Source: three-view drawing plus pictorial views. Frame: mm from the lowest corner of the part. Give positions to 0.01 mm unless a question says otherwise; leave off trailing zeros. Order: outer loops, then holes, each group sorted by start corner. A loop starts at its lowest first (then second) coordinate and runs counter-clockwise, first axis right, second up. Notation, with made-up numbers: (-35, 22.25) -> (-13, 22.25) arc R13 ccw to (-13, 44.25) -> close; hole circle Ø4 at (85, -25). An arc over 180 degrees is marked (long way). Answer in a Markdown table with one row per item. Add a question column.
Q1. Cut plane A-A on x = 894.5. Return the cut outline in (y, z), and give its area (3 significant figures).
Q2. Cut plane C-C on z = 46. Return the cut outline in (x, y).
Q3. Cut plane B-B on y = 720. Return the cut outline in (x, z), and give its area (3 significant figures).
Q4. Contact query for a flat-ended pin moving along its axis: P1, Ø24, axis at x = 641.5, z = 68, coming from the -Y side. Output: stop coordinate, or through.
Q5. Line query: line 1 along X through (y, z) = (712, 72.5); line 2 along Y through (x, z) = (908, 79); line 3 along X through (y, z) = (195, 59). Output: solid intervals per line, ascending. Write a range as from..to.
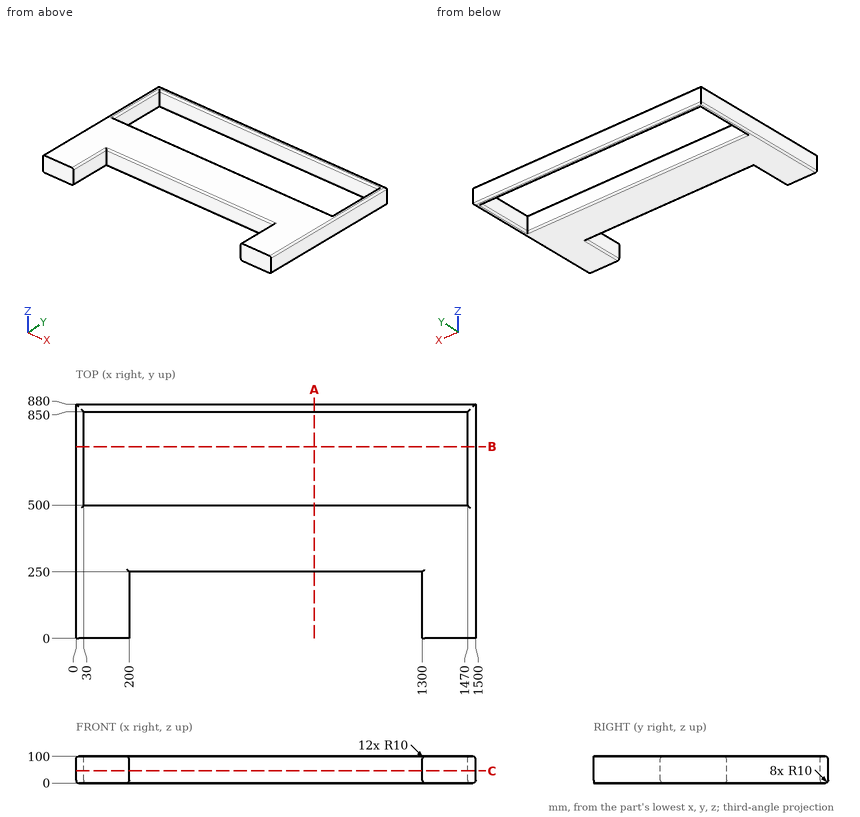
Completed:
| question | item | result |
|---|---|---|
| 1 | outline | (250, 10) arc R10 ccw to (260, 0) -> (490, 0) arc R10 ccw to (500, 10) -> (500, 90) arc R10 ccw to (490, 100) -> (260, 100) arc R10 ccw to (250, 90) -> close; (850, 10) arc R10 ccw to (860, 0) -> (870, 0) arc R10 ccw to (880, 10) -> (880, 90) arc R10 ccw to (870, 100) -> (860, 100) arc R10 ccw to (850, 90) -> close |
| 1 | area | 27,800 mm² |
| 2 | outline | (0, 0) -> (200, 0) -> (200, 250) -> (1300, 250) -> (1300, 0) -> (1500, 0) -> (1500, 880) -> (0, 880) -> close; hole (30, 500) -> (1470, 500) -> (1470, 850) -> (30, 850) -> close |
| 3 | outline | (0, 10) arc R10 ccw to (10, 0) -> (20, 0) arc R10 ccw to (30, 10) -> (30, 90) arc R10 ccw to (20, 100) -> (10, 100) arc R10 ccw to (0, 90) -> close; (1470, 10) arc R10 ccw to (1480, 0) -> (1490, 0) arc R10 ccw to (1500, 10) -> (1500, 90) arc R10 ccw to (1490, 100) -> (1480, 100) arc R10 ccw to (1470, 90) -> close |
| 3 | area | 5,830 mm² |
| 4 | P1 | stops at y = 250 |
| 5 | line 1 | x = 0..30, 1470..1500 |
| 5 | line 2 | y = 250..500, 850..880 |
| 5 | line 3 | x = 0..200, 1300..1500 |
